The figure shows three views and two pictorial views of one solid part (mm, origin at its lowest corner). Answer the questions. Round coordinates to 2 decimals unless told otherwise and drop trailing zeros. Order: outer loops, then holes, each group sorted by start corner. A loop starts at its lowest first (then second) coordinate and runs counter-clockwise, first axis right, second up. Notation, with made-up numbers: (28.5, 84.5) -> (61.5, 84.5) arc R25 ccw to (61.5, 101.5) -> close; hole circle Ø10 at (13, -17.75). An arc over 180 degrees is marked (long way). Answer as a JSON object with one key per item and string values. Group by question number.
Item 1: Section C-C, the plane y = 137.5 is taken. Write down the section's boundary in (x, z), plus the area to 3 significant figures.
Item 2: Section A-A, the plane y = 59 is taken. Write down the section's boundary in (x, z).
Item 3: Section B-B, the plane x = 20 is taken. Write down the section's boundary in (y, z), plus the area to 3 significant figures.
Item 4: Consider probe 1 along X at (y, z) = (137.5, 1.75); probe 2 along Y at (x, z) = (220, 2.7); probe 3 along Y at (x, z) = (20, 2.55). Determine where each line is inside the solid, lowest interval first. Write a range as from..to.
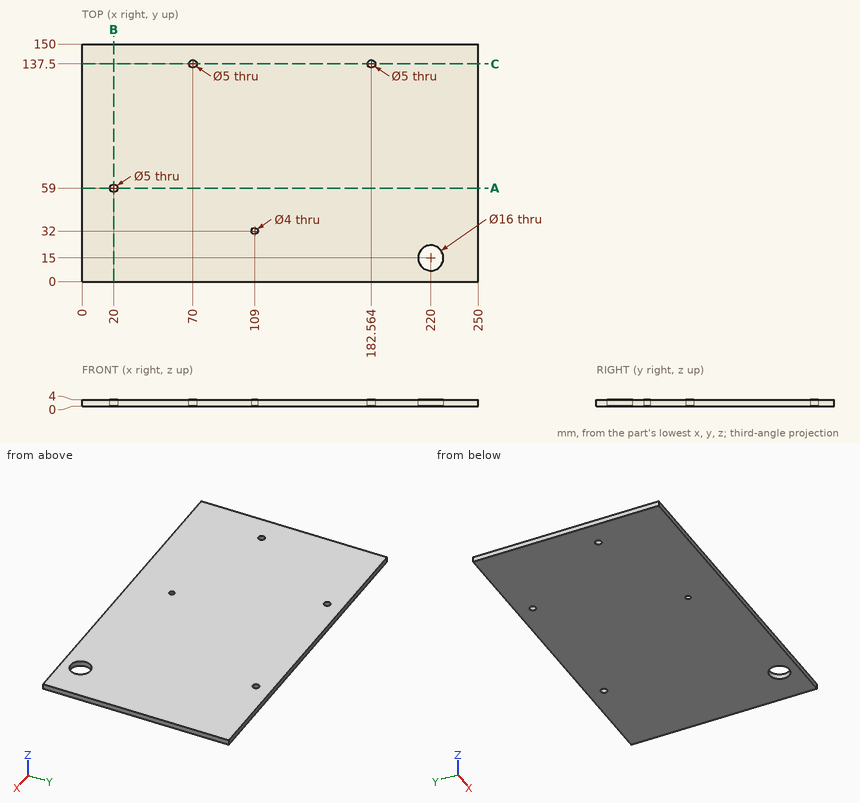
Values found:
{
 "1": {"outline": "(0, 0) -> (67.5, 0) -> (67.5, 4) -> (0, 4) -> close; (72.5, 0) -> (180.06, 0) -> (180.06, 4) -> (72.5, 4) -> close; (185.06, 0) -> (250, 0) -> (250, 4) -> (185.06, 4) -> close", "area": "960 mm2"},
 "2": {"outline": "(0, 0) -> (17.5, 0) -> (17.5, 4) -> (0, 4) -> close; (22.5, 0) -> (250, 0) -> (250, 4) -> (22.5, 4) -> close"},
 "3": {"outline": "(0, 0) -> (56.5, 0) -> (56.5, 4) -> (0, 4) -> close; (61.5, 0) -> (150, 0) -> (150, 4) -> (61.5, 4) -> close", "area": "580 mm2"},
 "4": {"probe 1": "0..67.5, 72.5..180.06, 185.06..250", "probe 2": "0..7, 23..150", "probe 3": "0..56.5, 61.5..150"}
}
